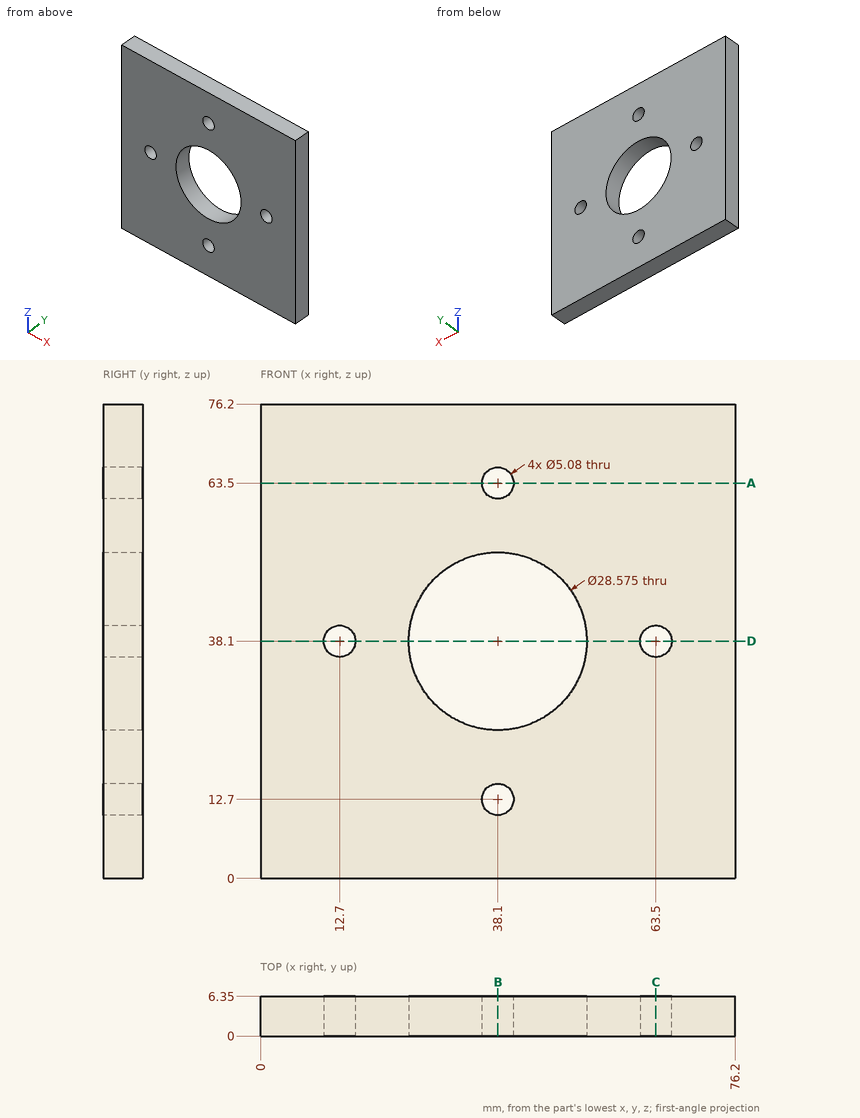
Geometry check sheet. Reference: drawing and pictorial views, mm from the part's lowest x, y, z. Give positions to 0.01 mm unless a question says otherwise; leave off trailing zeros. Loops run counter-clockwise (first coordinate to the right, second up) from the corner with the lowest first, then second, coordinate; pieces in that order, holes last. Notation, with made-up numbers: (67.5, 42.5) -> (90.5, 42.5) arc R26 cw to (90.5, 57.5) -> close; hole circle Ø7 at (-29.5, -16). An arc over 180 degrees is marked (long way). Answer in a Markdown table with one row per item. Add a question column.
1) Gauge pin test, flat end, axial feed: P1, Ø4, axis at x = 12.7, z = 38.1, coming from the +Y side. Record the tip position at first contact, or that the pin passes through.
2) Cross-section at D-D on z = 38.1. Record the boundary of the cut face in (x, y), and give its area (3 significant figures).
3) Material ranges on probe 1 along X at (y, z) = (3.5, 38.1); probe 2 along X at (y, z) = (1, 39); probe 3 along Z at (x, y) = (27.5, 2.75), recorded low to high. Write a range as from..to.
4) Cross-section at B-B on x = 38.1. Record the boundary of the cut face in (y, z).
5) Cross-section at A-A on z = 63.5. Record the boundary of the cut face in (x, y).
6) Cross-section at C-C on x = 63.5. Record the boundary of the cut face in (y, z).
Outcome:
| question | item | result |
|---|---|---|
| 1 | P1 | passes through |
| 2 | outline | (0, 0) -> (10.16, 0) -> (10.16, 6.35) -> (0, 6.35) -> close; (15.24, 0) -> (23.81, 0) -> (23.81, 6.35) -> (15.24, 6.35) -> close; (52.39, 0) -> (60.96, 0) -> (60.96, 6.35) -> (52.39, 6.35) -> close; (66.04, 0) -> (76.2, 0) -> (76.2, 6.35) -> (66.04, 6.35) -> close |
| 2 | area | 238 mm^2 |
| 3 | probe 1 | x = 0..10.16, 15.24..23.81, 52.39..60.96, 66.04..76.2 |
| 3 | probe 2 | x = 0..10.32, 15.08..23.84, 52.36..61.12, 65.88..76.2 |
| 3 | probe 3 | z = 0..28.52, 47.68..76.2 |
| 4 | outline | (0, 0) -> (6.35, 0) -> (6.35, 10.16) -> (0, 10.16) -> close; (0, 15.24) -> (6.35, 15.24) -> (6.35, 23.81) -> (0, 23.81) -> close; (0, 52.39) -> (6.35, 52.39) -> (6.35, 60.96) -> (0, 60.96) -> close; (0, 66.04) -> (6.35, 66.04) -> (6.35, 76.2) -> (0, 76.2) -> close |
| 5 | outline | (0, 0) -> (35.56, 0) -> (35.56, 6.35) -> (0, 6.35) -> close; (40.64, 0) -> (76.2, 0) -> (76.2, 6.35) -> (40.64, 6.35) -> close |
| 6 | outline | (0, 0) -> (6.35, 0) -> (6.35, 35.56) -> (0, 35.56) -> close; (0, 40.64) -> (6.35, 40.64) -> (6.35, 76.2) -> (0, 76.2) -> close |
